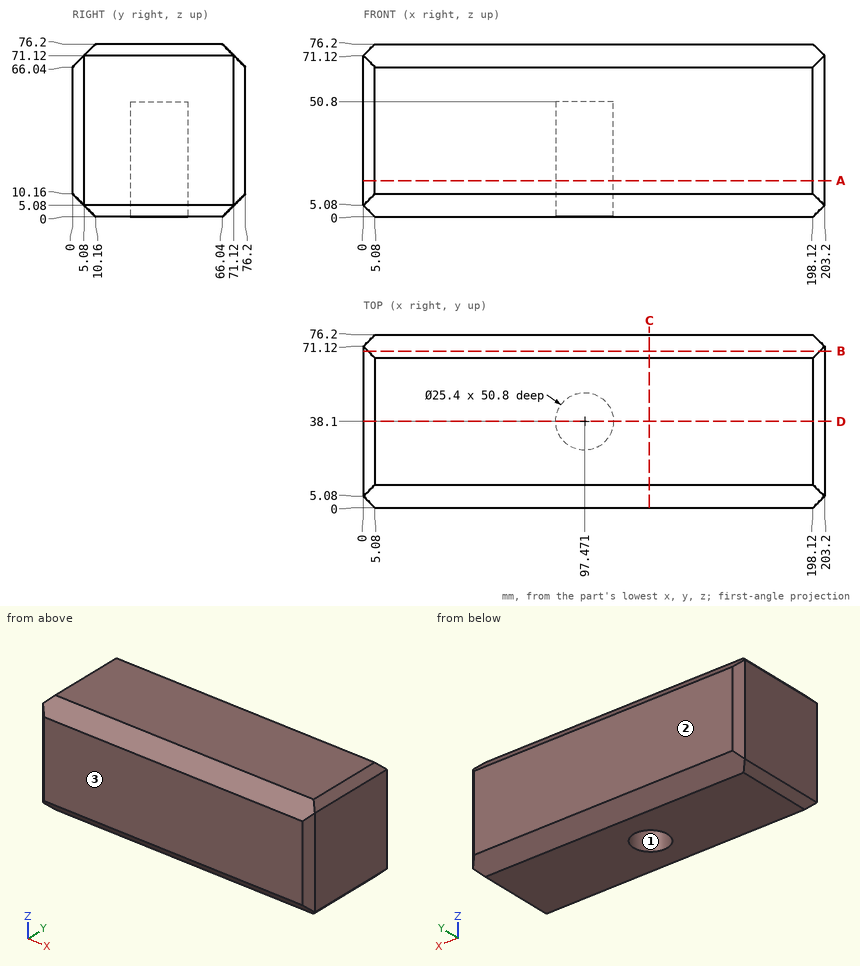
Geometry check sheet. Reference: drawing and pictorial views, mm from the part's lowest x, y, z. Give positions to 0.01 mm unless a question says otherwise; leave off trailing zeros. Write each loop counter-clockwise with the first axis right and the second up, starting at its lowest first coordinate (ties: lowest second). Pieces come first, ordered by that corner, then holes. Notation, with made-up numbers: (6.25, 75) -> (41.25, 75) arc R26 ccw to (41.25, 110) -> close; hole circle Ø11 at (-7, 60). An arc over 180 degrees is marked (long way). One line per item, written item: value. Start each with the question number.
Item 1: Section check B-B on y = 69. Record the cut outline in (x, z), then the cut area to 3 significant figures.
Item 2: Draft check along Y on the marked faces 1, 2 and 3. Enter one of: +Y half, -Y half, draft (parallel to the pull), parting line (faces both ways), or undercut.
Item 3: Gauge pin test, flat end, axial feed: pin 1 (20.5 mm diameter, centred on x = 97.47, y = 38.1, fed in from -Z). Record the tip position at first contact, or that the pin passes through.
Item 4: Section check D-D on y = 38.1. Record the cut outline in (x, z).
Item 5: Section check A-A on z = 16. Record the cut outline in (x, y).
Item 6: Section check C-C on x = 126. Record the cut outline in (y, z), then the cut area to 3 significant figures.
Item 7: Material ranges on probe 1 along X at (y, z) = (38, 32); probe 2 along X at (y, z) = (37, 29); probe 3 along Y at (x, z) = (39, 70.5), recorded low to high. Write a range as from..to.
Results list:
1. outline: (0, 5.08) -> (2.12, 2.96) -> (201.08, 2.96) -> (203.2, 5.08) -> (203.2, 71.12) -> (201.08, 73.24) -> (2.12, 73.24) -> (0, 71.12) -> close
1. area: 14,300 mm²
2. face 1: undercut
2. face 2: +Y half
2. face 3: -Y half
3. pin 1: z = 50.8
4. outline: (0, 5.08) -> (5.08, 0) -> (84.77, 0) -> (84.77, 50.8) -> (110.17, 50.8) -> (110.17, 0) -> (198.12, 0) -> (203.2, 5.08) -> (203.2, 71.12) -> (198.12, 76.2) -> (5.08, 76.2) -> (0, 71.12) -> close
5. outline: (0, 5.08) -> (5.08, 0) -> (198.12, 0) -> (203.2, 5.08) -> (203.2, 71.12) -> (198.12, 76.2) -> (5.08, 76.2) -> (0, 71.12) -> close; hole circle Ø25.4 at (97.47, 38.1)
6. outline: (0, 10.16) -> (10.16, 0) -> (66.04, 0) -> (76.2, 10.16) -> (76.2, 66.04) -> (66.04, 76.2) -> (10.16, 76.2) -> (0, 66.04) -> close
6. area: 5,600 mm²
7. probe 1: 0..84.77, 110.17..203.2
7. probe 2: 0..84.82, 110.12..203.2
7. probe 3: 4.46..71.74
